The model under review builds one solid part; all positions refer to its coordinate system, in mm. A direction names the side the tool comes from. Coordinates: 2 decimals unless noted, no trailing zeros. Loops run counter-clockwise (first coordinate to the right, second up) from the corner with the lowest first, then second, coordinate; pieces in that order, holes last. Notation, with made-up numbers: M 9.25,42 L 23.25,42 A11 ccw 23.25,50 Z; hole C -10,-27.5 d3. An arc over 180 degrees is marked long. Write item = value, one per line. Start each with the question number.
Q1. We need section B-B on x = -73.5. Give the boundary of the cut face in (y, z), and give its area (3 significant figures).
Q2. Mouldability with a two-part tool opening along X and no side actions: class faces 3 (the face through (-90, -19, -10)), 4 (the face through (-91.972, -32.441, -13.802)), 5 (the face through (-94, -19, -7)), 6 (the face through (-73.092, -8.774, 2.028)) as released by +X, released by -X, zero draft, split by the parting line, or undercut.
Q3. For faces 1 (the face through (-80, -24, 0)), 2 (the face through (-70, -9, 2)), list the 3-axis set-ups (+Z, -Z, +X, -X, +Y, -Y) from which the entire face can be reached by the end or side of a thin tool; tool diameter is ignored.
Q4. Wall thickness on probe 1 along Y at (x, z) = (-75, 0.95) (3 decimals); probe 2 along Z at (x, y) = (-75.25, -13.5); probe 3 along X at (y, z) = (-25, -16): over which ranges is each line inside the solid? List them lowest first.
Q5. We need section C-C on y = -15.5. Give the boundary of the cut face in (x, z).
Q6. We need section D-D on x = -92. Give the boundary of the cut face in (y, z) (3 decimals).
Q7. Clearance check with flat-ended pins moving along their axes: pin 1 Ø5 at (y, z) = (-9.375, -20) entering from +X; pin 2 Ø6 at (y, z) = (-32, -0.5) entering from +X; pin 3 Ø6 at (x, y) = (-81, -29) entering from -Z. State where each tip first meets the part, or that it passes through.
Q8. We need section A-A on z = -20. Give the boundary of the cut face in (x, y) (3 decimals), and give its area (3 significant figures).
from build123d import *

# Parameters (mm, degrees)
BOSS_EXTRUDE1_DEPTH = 4
BOSS_EXTRUDE2_DEPTH = 4
CUT_EXTRUDE1_DEPTH  = 111.599740054
SKETCH4_R           = 2
CUT_EXTRUDE2_DEPTH  = 4
SKETCH5_R           = 2
CUT_EXTRUDE3_DEPTH  = 4


with BuildPart() as part:
    # Sketch1 → Boss-Extrude1 (new body)
    with BuildSketch(Plane.XY):
        Polygon((-90, -50.55), (-75, -50.55), (-70, -17.75), (-70, -1), (-80, -1), (-90, -1), (-90, -17.75), align=None)
    extrude(amount=BOSS_EXTRUDE1_DEPTH)

    # Sketch2 → Boss-Extrude2 (add)
    with BuildSketch(Plane.ZY.offset(90)):
        Polygon((0, -1), (-25, -1), (-25, -17.75), (0, -50.55), (4, -50.55), (4, -1), align=None)
    extrude(amount=BOSS_EXTRUDE2_DEPTH)

    # Sketch3 → Cut-Extrude1 (cut, through all)
    with BuildSketch(Plane.XY.offset(4)):
        Polygon((-94, -49.55), (-94, -50.55), (-75, -50.55), (-74.542682927, -47.55), (-94, -47.55), align=None)
    extrude(amount=-CUT_EXTRUDE1_DEPTH, mode=Mode.SUBTRACT)

    # Sketch4 → Cut-Extrude2 (cut)
    with BuildSketch(Plane.XY.offset(4)):
        with Locations((-75, -9.375)):
            Circle(SKETCH4_R)
    extrude(amount=-CUT_EXTRUDE2_DEPTH, mode=Mode.SUBTRACT)

    # Sketch5 → Cut-Extrude3 (cut)
    with BuildSketch(Plane.ZY.offset(94)):
        with Locations((-20, -9.375)):
            Circle(SKETCH5_R)
    extrude(amount=-CUT_EXTRUDE3_DEPTH, mode=Mode.SUBTRACT)


solid = part.part
Returned:
q1.outline = M -40.71,0 L -10.7,0 L -10.7,4 L -40.71,4 Z; M -8.05,0 L -1,0 L -1,4 L -8.05,4 Z
q1.area = 148 mm^2
q2.face_3 = released by +X
q2.face_4 = zero draft
q2.face_5 = released by -X
q2.face_6 = undercut
q3.face_1 = -Z, +X, +Y, -Y
q3.face_2 = +Z, -Z, +X, +Y, -Y
q4.probe_1 = -47.55 to -11.375, -7.375 to -1
q4.probe_2 = 0 to 4
q4.probe_3 = -94 to -90
q5.outline = M -94,-25 L -90,-25 L -90,0 L -70,0 L -70,4 L -94,4 Z
q6.outline = M -47.55,-2.287 L -17.75,-25 L -1,-25 L -1,4 L -47.55,4 Z; hole C -9.375,-20 d4
q7.pin_1 = -90
q7.pin_2 = -71.72
q7.pin_3 = 0
q8.outline = M -94,-24.31 L -90,-24.31 L -90,-11.375 L -94,-11.375 Z; M -94,-7.375 L -90,-7.375 L -90,-1 L -94,-1 Z
q8.area = 77.2 mm^2
